Geometry: final body of the model. Coordinates: model frame, mm. Face numbers are marked on the shaded views. A direction names the side the tool comes from. Give positions to 0.01 mm unless a question says otherwise; leave off trailing zeros. Order: outer loops, then holes, each group sorted by start corner. A loop starts at its lowest first (then second) coordinate and runs counter-clockwise, first axis right, second up. Notation, with made-up numbers: (83, 83.25) - (123, 83.25) arc R5 cw to (123, 87.25) - close; hole circle Ø6 at (33, 3.5). An arc over 180 degrees is marked (long way). Put each result on its own line as item: value. Start each with the question number.
1. Section B-B on x = 20.5. Return the cut outline in (y, z), plus the area to 3 significant figures.
2. Section A-A on z = -19. Return the cut outline in (x, y), plus the area to 3 significant figures.
3. Set-up query: the marked faces 1, 2 and 3. Return all of +Z, -Z, +X, -X, +Y, -Y with unobstructed straight access to the full face (end or side cutting, diameter ignored); none if empty.
4. Ray query, line 1 along Z through (x, y) = (1.6, 5); line 2 along Y through (x, z) = (1.15, 39.45); line 3 along Y through (x, z) = (-1, 39). Return the intervals inside material, ascending. Write a range as from..to.
5. First-contact query: P1, Ø6, axis at y = 7, z = -15.5, coming from the +X side; P2, Ø4, axis at x = -25, z = 2, coming from the +Y side; P3, Ø6, axis at y = 8, z = -9, coming from the -X side. Flat tips, straight axial feed; report the tip coordinate or a pass-through.
Solid Edge part; units mm, degrees
sketch "Sketch1" plane through (0, 0, 0) normal (0, -1, 0) x (1, 0, 0)
  arc A0 (235.56, 35.1) -> (235.56, 41.1) centre (235.56, 38.1) ccw
  line L0 (229.56, 41.1) -> (235.56, 41.1)
  arc A1 (229.56, 41.1) -> (229.56, 35.1) centre (229.56, 38.1) ccw
  line L1 (235.56, 35.1) -> (229.56, 35.1)
  arc A2 (-235.56, -35.1) -> (-235.56, -41.1) centre (-235.56, -38.1) ccw
  line L2 (-229.56, -41.1) -> (-235.56, -41.1)
  arc A3 (-229.56, -41.1) -> (-229.56, -35.1) centre (-229.56, -38.1) ccw
  line L3 (-235.56, -35.1) -> (-229.56, -35.1)
  line L4 (-241.3, -44.45) -> (-241.3, 44.45)
  line L5 (-241.3, 44.45) -> (241.3, 44.45)
  line L6 (241.3, 44.45) -> (241.3, -44.45)
  line L7 (241.3, -44.45) -> (-241.3, -44.45)
  line L8 (235.56, -35.1) -> (229.56, -35.1)
  arc A4 (229.56, -41.1) -> (229.56, -35.1) centre (229.56, -38.1) cw
  line L9 (229.56, -41.1) -> (235.56, -41.1)
  arc A5 (235.56, -35.1) -> (235.56, -41.1) centre (235.56, -38.1) cw
  line L10 (-235.56, 35.1) -> (-229.56, 35.1)
  arc A6 (-229.56, 41.1) -> (-229.56, 35.1) centre (-229.56, 38.1) cw
  line L11 (-229.56, 41.1) -> (-235.56, 41.1)
  arc A7 (-235.56, 35.1) -> (-235.56, 41.1) centre (-235.56, 38.1) cw
extrude "Protrusion1" add sketch "Sketch1" along normal blind 3
sketch "Sketch2" plane through (0, -3, 0) normal (0, -1, 0) x (1, 0, 0)
  line L0 (0, 44.45) -> (-3, 44.45)
  line L1 (-3, 44.45) -> (-3, -44.45)
  line L2 (-3, -44.45) -> (0, -44.45)
  line L3 (0, -44.45) -> (3, -44.45)
  line L4 (3, -44.45) -> (3, 44.45)
  line L5 (3, 44.45) -> (0, 44.45)
extrude "RackPlateDivider" add sketch "Sketch2" against normal blind 13
hole "Hole1" at (3, 5, 39.45) direction (-1, 0, 0) diameter 4 end up to next
hole "Hole2" at (3, 5, -39.45) direction (-1, 0, 0) diameter 4 end up to next
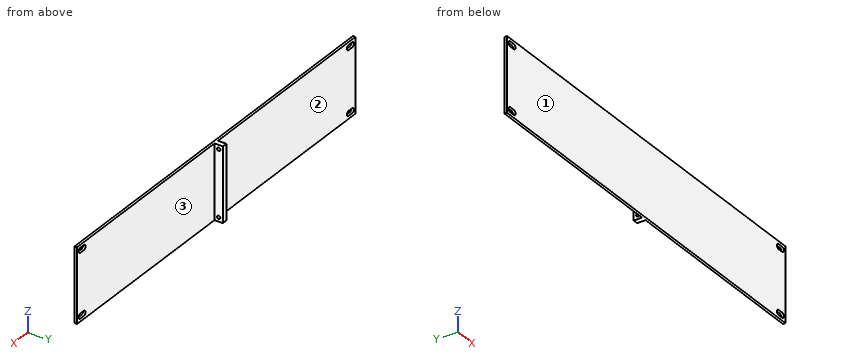
Resolved:
1. outline: (-3, -44.45) - (0, -44.45) - (0, 44.45) - (-3, 44.45) - close
1. area: 267 mm^2
2. outline: (-241.3, -3) - (241.3, -3) - (241.3, 0) - (3, 0) - (3, 10) - (-3, 10) - (-3, 0) - (-241.3, 0) - close
2. area: 1,510 mm^2
3. face 1: +Z, -Z, +X, -X, -Y
3. face 2: +Z, -Z, -X, +Y
3. face 3: +Z, -Z, +X, +Y
4. line 1: -44.45..-41.45, -37.45..37.45, 41.45..44.45
4. line 2: -3..3, 7..10
4. line 3: -3..3.05, 6.95..10
5. P1: x = 3
5. P2: y = 0
5. P3: x = -3
